Here's how the part is built. I have some questions about the finished solid (model axes, mm). Face numbers are marked on the shaded views. A direction names the side the tool comes from. Round coordinates to 2 decimals unless told otherwise and drop trailing zeros. Order: outer loops, then holes, each group sorted by start corner. A loop starts at its lowest first (then second) coordinate and runs counter-clockwise, first axis right, second up. Notation, with made-up numbers: (0.5, -18) -> (39.5, -18) arc R34 ccw to (39.5, 15) -> close; hole circle Ø6 at (-13.5, 17). An arc over 180 degrees is marked (long way). Answer in a Markdown table with one row per item.
```python
from build123d import *

# Parameters (mm, degrees)
BOSS_EXTRUDE1_DEPTH = 11.7983
SKETCH2_W           = 2.782556626
SKETCH2_H           = 16.695339754
CUT_EXTRUDE1_DEPTH  = 39.088832947
CHAMFER5_SIZE       = 0.635
FILLET1_R           = 0.635
SKETCH3_W           = 12.446
SKETCH3_H           = 11.938
CUT_EXTRUDE2_DEPTH  = 23.5966
CUT_EXTRUDE3_DEPTH  = 23.5966
CUT_EXTRUDE4_DEPTH  = 12.446


with BuildPart() as part:
    # Sketch1 → Boss-Extrude1 (new, symmetric)
    with BuildSketch(Plane.XY):
        with BuildLine():
            Line((0, 0), (9.1948, 0))
            ThreePointArc((9.1948, 0), (9.917795425, 2.47592173), (12.065820738, 3.903821604))
            ThreePointArc((12.065820738, 3.903821604), (12.561454562, 3.97266008), (13.060965958, 3.942995467))
            Line((13.060965958, 3.942995467), (26.333208305, 1.828629586))
            ThreePointArc((26.333208305, 1.828629586), (27.918052264, 2.09049066), (29.028861508, 3.25083734))
            ThreePointArc((29.028861508, 3.25083734), (29.318103156, 4.275095808), (29.256355961, 5.337618007))
            ThreePointArc((29.256355961, 5.337618007), (28.148880761, 6.911407154), (26.255762963, 7.25697712))
            ThreePointArc((26.255762963, 7.25697712), (24.102846991, 7.114861278), (21.9964, 7.5819))
            Line((21.9964, 7.5819), (21.9964, 13.0937))
            ThreePointArc((21.9964, 13.0937), (21.624425612, 13.991725612), (20.7264, 14.3637))
            Line((20.7264, 14.3637), (14.8336, 14.3637))
            ThreePointArc((14.8336, 14.3637), (13.935574388, 14.735674388), (13.5636, 15.6337))
            Line((13.5636, 15.6337), (13.5636, 18.6944))
            Line((13.5636, 18.6944), (5.08, 21.2344))
            ThreePointArc((5.08, 21.2344), (1.287669396, 10.916800623), (0, 0))
        make_face()
    extrude(amount=BOSS_EXTRUDE1_DEPTH, both=True)

    # Sketch2 → Cut-Extrude1 (cut, through all)
    with BuildSketch(Plane(origin=(0, 0, 0), x_dir=(0, 0, -1), z_dir=(1, 0, 0))):
        with Locations((-10.878178313, 17.707569877)):
            Rectangle(SKETCH2_W, SKETCH2_H)
        with Locations((10.878178313, 17.707569877)):
            Rectangle(SKETCH2_W, SKETCH2_H)
    extrude(amount=CUT_EXTRUDE1_DEPTH, mode=Mode.SUBTRACT)

    # Chamfer5
    # the kernel refuses this chamfer: 0.635 mm, written as the material it takes off along each edge
    with BuildSketch(Plane(origin=(22.359418697, 14.3637, 9.4869), x_dir=(0, -0.9996219169112966, 0.02749587661058734), z_dir=(-1, 0, 0))) as chamfer5_piece_1:
        Polygon((CHAMFER5_SIZE * 0.999621916911, -CHAMFER5_SIZE * 0.0274958766106), (-CHAMFER5_SIZE * 0.0274958766106, -CHAMFER5_SIZE * 0.999621916911), (0, 0), align=None)
    extrude(amount=7.525818697, mode=Mode.SUBTRACT)
    with BuildSketch(Plane(origin=(14.8336, 15.6337, 9.4869), x_dir=(-1, 0, 0), z_dir=(0, 1, 0))) as chamfer5_piece_2:
        Polygon((1.27 + CHAMFER5_SIZE, 0), (1.27, -CHAMFER5_SIZE), (1.27, 0), align=None)
    revolve(axis=Axis((14.8336, 15.6337, 9.4869), (0, 0, 1)), revolution_arc=90, mode=Mode.SUBTRACT)
    with BuildSketch(Plane(origin=(13.5636, 15.6337, 9.4869), x_dir=(-0.9996219169112968, 0, 0.02749587661058727), z_dir=(0, 1, 0))) as chamfer5_piece_3:
        Polygon((CHAMFER5_SIZE * 0.999621916911, -CHAMFER5_SIZE * 0.0274958766106), (-CHAMFER5_SIZE * 0.0274958766106, -CHAMFER5_SIZE * 0.999621916911), (0, 0), align=None)
    extrude(amount=4.693718697, mode=Mode.SUBTRACT)
    with BuildSketch(Plane(origin=(13.5636, 15.6337, -9.4869), x_dir=(-0.9996219169112968, 0, -0.02749587661058727), z_dir=(0, 1, 0))) as chamfer5_piece_4:
        Polygon((CHAMFER5_SIZE * 0.999621916911, CHAMFER5_SIZE * 0.0274958766106), (-CHAMFER5_SIZE * 0.0274958766106, CHAMFER5_SIZE * 0.999621916911), (0, 0), align=None)
    extrude(amount=4.693718697, mode=Mode.SUBTRACT)
    with BuildSketch(Plane(origin=(14.8336, 15.6337, -9.4869), x_dir=(-1, 0, 0), z_dir=(0, 1, 0))) as chamfer5_piece_5:
        Polygon((1.27 + CHAMFER5_SIZE, 0), (1.27, CHAMFER5_SIZE), (1.27, 0), align=None)
    revolve(axis=Axis((14.8336, 15.6337, -9.4869), (0, 0, 1)), revolution_arc=90, mode=Mode.SUBTRACT)
    with BuildSketch(Plane(origin=(22.359418697, 14.3637, -9.4869), x_dir=(0, -0.9996219169112968, -0.027495876610587194), z_dir=(-1, 0, 0))) as chamfer5_piece_6:
        Polygon((CHAMFER5_SIZE * 0.999621916911, CHAMFER5_SIZE * 0.0274958766106), (-CHAMFER5_SIZE * 0.0274958766106, CHAMFER5_SIZE * 0.999621916911), (0, 0), align=None)
    extrude(amount=7.525818697, mode=Mode.SUBTRACT)

    # Fillet1
    fillet1_edges = [part.edges().sort_by_distance(p)[0] for p in [
        (5.08, 21.2344, 0),
    ]]
    fillet(fillet1_edges, radius=FILLET1_R)

    # Sketch3 → Cut-Extrude2 (cut)
    with BuildSketch(Plane(origin=(0, 0, 0), x_dir=(0, 0, -1), z_dir=(1, 0, 0))):
        with Locations((0, 5.969)):
            Rectangle(SKETCH3_W, SKETCH3_H)
    extrude(amount=CUT_EXTRUDE2_DEPTH, mode=Mode.SUBTRACT)

    # Sketch4 → Cut-Extrude3 (cut)
    with BuildSketch(Plane(origin=(0, 11.938, 0), x_dir=(-1, 0, 0), z_dir=(0, -1, 0))):
        with BuildLine():
            Line((-18.943995478, -6.223), (-24.384, -6.223))
            Line((-24.384, -6.223), (-24.384, -6.35))
            ThreePointArc((-24.384, -6.35), (-24.755974388, -7.248025612), (-25.654, -7.62))
            Line((-25.654, -7.62), (-29.337, -7.62))
            Line((-29.337, -7.62), (-29.337, 7.62))
            Line((-29.337, 7.62), (-25.654, 7.62))
            ThreePointArc((-25.654, 7.62), (-24.755974388, 7.248025612), (-24.384, 6.35))
            Line((-24.384, 6.35), (-24.384, 6.223))
            Line((-24.384, 6.223), (-18.943995478, 6.223))
            Line((-18.943995478, 6.223), (-18.943995478, -6.223))
        make_face()
    extrude(amount=CUT_EXTRUDE3_DEPTH, mode=Mode.SUBTRACT)

    # Sketch5 → Cut-Extrude4 (cut)
    with BuildSketch(Plane.XY.offset(-6.223)):
        Polygon((17.373606876, 11.930026708), (4.9022, 14.705176479), (4.267958712, 19.552209242), (1.539127618, 19.552209242), (1.539127618, 11.930026708), align=None)
    extrude(amount=CUT_EXTRUDE4_DEPTH, mode=Mode.SUBTRACT)


solid = part.part
```
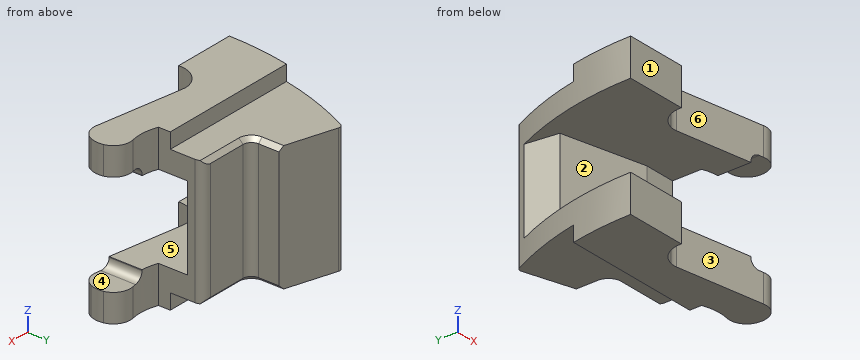
1. For pin 1 Ø1.2 at (x, z) = (6.5, 11) entering from +Y; pin 2 Ø1.4 at (x, z) = (20, 1) entering from -Y; pin 3 Ø1 at (x, z) = (24, -6.5) entering from -Y, each with a flat end and sliding along its axis, tell me the tip position at first contact or that it passes through.
Numbers:
| item | result |
|---|---|
| pin 1 | stops at y = 9.36 |
| pin 2 | stops at y = 11.94 |
| pin 3 | stops at y = 2.13 |
2. Suppose I cut it at B-B on x = 27.5. Write out the boundary of the cut face in (y, z), then the cut area to 3 significant figures.
Numbers:
| item | result |
|---|---|
| outline | (1.92, -11.8) -> (7.21, -11.8) -> (7.21, -7.62) -> (1.92, -7.62) -> close; (1.92, 7.62) -> (7.21, 7.62) -> (7.21, 11.8) -> (1.92, 11.8) -> close |
| area | 44.2 mm2 |
3. For the marked faces 4, 5 and 6, which set-ups out of +Z, -Z, +X, -X, +Y, -Y let a thin tool reach every point of the face, with its end or its side?
Numbers:
| item | result |
|---|---|
| face 4 | +X, +Y, -Y |
| face 5 | -X, -Y |
| face 6 | +Z, -Z, -Y |
4. Suppose I cut it at D-D on y = 17.5. Write out the boundary of the cut face in (x, z), then the cut area to 3 significant figures.
Numbers:
| item | result |
|---|---|
| outline | (3.39, -9.49) -> (12.93, -9.49) -> (13.56, -8.85) -> (13.56, 8.85) -> (12.93, 9.49) -> (3.39, 9.49) -> (3.39, 6.22) -> (4.54, 6.22) -> (4.54, -6.22) -> (3.39, -6.22) -> close |
| area | 178 mm2 |
5. Suppose I cut it at A-A on z = 4.25. Write out the boundary of the cut face in (x, y) (3 decimals), then the cut area to 3 significant figures.
Numbers:
| item | result |
|---|---|
| outline | (4.268, 19.552) -> (4.902, 14.705) -> (17.338, 11.938) -> (21.996, 11.938) -> (21.996, 13.094) arc R1.27 ccw to (20.726, 14.364) -> (14.834, 14.364) arc R1.27 cw to (13.564, 15.634) -> (13.564, 18.694) -> (5.591, 21.081) arc R0.635 ccw to (4.84, 20.754) arc R46.92 ccw to start |
| area | 74.9 mm2 |
6. We'd pull the mould along X, two halves only. Please class the marked faces 1, 2 and 3: released by +X, released by -X, zero draft, split by the parting line, or undercut.
Numbers:
| item | result |
|---|---|
| face 1 | zero draft |
| face 2 | released by -X |
| face 3 | undercut |
7. Please list where these lines run through material, in increasing order: line 1 along Z through (x, y) = (16.75, 6.75); line 2 along Z through (x, y) = (9, 10.5); line 3 along Y through (x, z) = (5, 10.25).
Numbers:
| item | result |
|---|---|
| line 1 | z = -11.8 to -6.22, 6.22 to 11.8 |
| line 2 | z = -9.49 to -6.22, 6.22 to 9.49 |
| line 3 | y = 0 to 9.36 |
8. Suppose I cut it at C-C on y = 8.5. Write out the boundary of the cut face in (x, z).
Numbers:
| item | result |
|---|---|
| outline | (0.78, -11.8) -> (22, -11.8) -> (22, -6.22) -> (0.78, -6.22) -> close; (0.78, 6.22) -> (22, 6.22) -> (22, 11.8) -> (0.78, 11.8) -> close |
